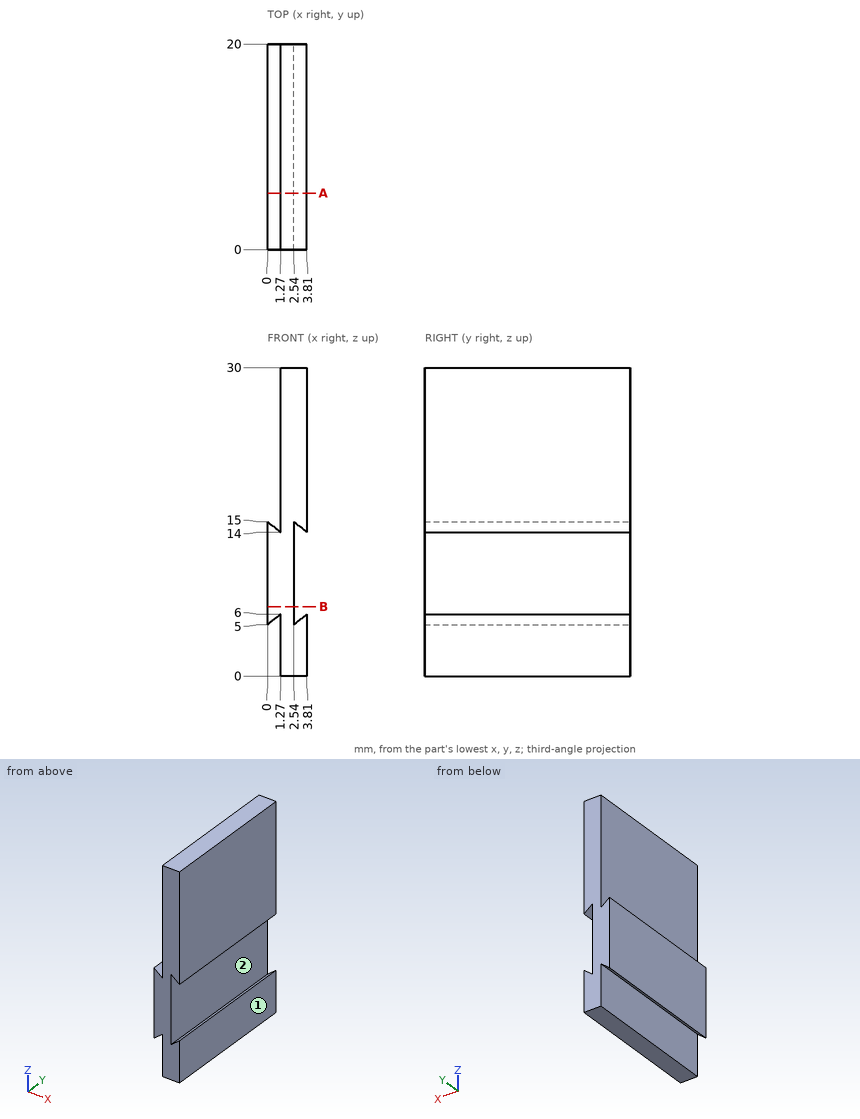
Study the drawing (mm; zero at the part's minimum x, y, z) and answer. Give positions to 0.01 mm unless a question says otherwise; leave off trailing zeros. Loops run counter-clockwise (first coordinate to the right, second up) from the corner with the lowest first, then second, coordinate; pieces in that order, holes last. Notation, with made-up numbers: (-26, 64.25) -> (6, 64.25) arc R20 cw to (6, 94.25) -> close; hole circle Ø7 at (-22.75, -15.75). An arc over 180 degrees is marked (long way). Use a Markdown table: item, result. Add a question column.
1) Each of these flat-tipped pins is pushed along its axis until it touches: P1, Ø5, axis at y = 13, z = 22, coming from the -X side; P2, Ø3, axis at y = 12, z = 10, coming from the +X side. Where does it stop, or does it pass through?
2) For a pull along Z with two mould halves and no side action, classify the marked faces 1 and 2 as +Z half, -Z half, draft (parallel to the pull), parting line (faces both ways), or undercut.
3) Consider line 1 along X through (y, z) = (3.5, 8.75); line 2 along X through (y, z) = (11.75, 25.5); line 3 along Z through (x, y) = (2.7, 4.25). Determine where each line is inside the solid, lowest interval first.
4) The part is cut by section A-A, the plane y = 5.5. Determine the outline of the cut face in (x, z).
5) The part is cut by section B-B, the plane z = 6.75. Determine the outline of the cut face in (x, y), plus the area to 3 significant figures.
Reported:
| question | item | result |
|---|---|---|
| 1 | P1 | stops at x = 1.27 |
| 1 | P2 | stops at x = 2.54 |
| 2 | face 1 | draft |
| 2 | face 2 | undercut |
| 3 | line 1 | x = 0 to 2.54 |
| 3 | line 2 | x = 1.27 to 3.81 |
| 3 | line 3 | z = 0 to 5.13, 14.87 to 30 |
| 4 | outline | (0, 5) -> (1.27, 6) -> (1.27, 0) -> (3.81, 0) -> (3.81, 6) -> (2.54, 5) -> (2.54, 15) -> (3.81, 14) -> (3.81, 30) -> (1.27, 30) -> (1.27, 14) -> (0, 15) -> close |
| 5 | outline | (0, 0) -> (2.54, 0) -> (2.54, 20) -> (0, 20) -> close |
| 5 | area | 50.8 mm^2 |
